Check sheet for the modelled part. Datum: model origin and axes. Units: mm. Give positions to 0.01 mm unless a question says otherwise; leave off trailing zeros. Loops run counter-clockwise (first coordinate to the right, second up) from the corner with the lowest first, then second, coordinate; pieces in that order, holes last. Notation, with made-up numbers: M 22,11.5 L 60,11.5 A10 cw 60,24.5 Z; hole C 26.5,-27 d8. An arc over 180 degrees is marked long. Write each question's results on one line, items separated by ' | '. Start each with the question number.
1. Sectioned sample at C-C on z = 40.64. Record the cut outline in (x, y).
2. Material ranges on line 1 along X through (y, z) = (1.6, 20.32) (3 decimals); line 2 along Z through (x, y) = (1, 4.25); line 3 along X through (y, z) = (2.5, -22) (3 decimals), recorded low to high.
3. Sectioned sample at B-B on y = 1. Record the cut outline in (x, z) (3 decimals), and give its area (3 significant figures).
4. Draft check along Z on faces 1 (the flat face through (-4.696, 3.131, -48.988)), 2 (the cylindrical face through (-2.435, 2.164, -0.767)), 3 (the cylindrical face through (0.553, 2.164, -38.148)), 4 (the flat face through (-4, 0, -1)). Enter one of: pulls with the +Z half, pulls with the -Z half, needs draft (parallel to the pull), parting line crosses it, or undercut.
5. Go/stop test with flat-tipped pins: pin 1 (1 mm diameter, centred on x = 2.5, y = 4, fed in from -Z); pin 2 (1 mm diameter, centred on x = 6, y = 5.5, fed in from -Z). Record where each tip stops, or that it passes through.
6. Sectioned sample at D-D on x = -1. Give the number of separate pieces and of enclosed holes in the cut face, and give its area (3 significant figures).
```python
from build123d import *

# Parameters (mm, degrees)
BOSS_EXTRUDE1_DEPTH                                = 6.35
CSK_FOR_10_FLAT_HEAD_MACHINE_SCREW_100_D           = 5.1054
CSK_FOR_10_FLAT_HEAD_MACHINE_SCREW_100_CSINK_D     = 9.779
CSK_FOR_10_FLAT_HEAD_MACHINE_SCREW_100_CSINK_ANGLE = 100


with BuildPart() as part:
    # Sketch1 → Boss-Extrude1 (new body)
    with BuildSketch(Plane(origin=(0, 0, 0), x_dir=(1, 0, 0), z_dir=(0, 1, 0))):
        Polygon((0, 60.325), (-9.525, 37.329615818), (-9.525, -37.329615818), (0, -60.325), (9.525, -37.329615818), (9.525, 37.329615818), align=None)
    extrude(amount=BOSS_EXTRUDE1_DEPTH)

    # CSK for #10 Flat Head Machine Screw (100)1 (through all)
    with Locations(Plane(origin=(0, 6.35, 0), x_dir=(1, 0, 0), z_dir=(0, 1, 0))):
        with Locations((0, 20.32), (0, 40.64), (0, 0), (0, -20.32), (0, -40.64)):
            CounterSinkHole(CSK_FOR_10_FLAT_HEAD_MACHINE_SCREW_100_D / 2, CSK_FOR_10_FLAT_HEAD_MACHINE_SCREW_100_CSINK_D / 2, counter_sink_angle=CSK_FOR_10_FLAT_HEAD_MACHINE_SCREW_100_CSINK_ANGLE)


solid = part.part
```
Output values:
1) outline: M -8.15,0 L -2.55,0 L -2.55,4.39 L -4.89,6.35 L -8.15,6.35 Z; M 2.55,0 L 8.15,0 L 8.15,6.35 L 4.89,6.35 L 2.55,4.39 Z
2) line 1: -9.525 to -2.553, 2.553 to 9.525 | line 2: -57.91 to -42.99, -38.29 to -22.67, -17.97 to -2.35, 2.35 to 17.97, 22.67 to 38.29, 42.99 to 57.91 | line 3: -9.525 to -1.922, 1.922 to 9.525
3) outline: M -9.525,-37.33 L 0,-60.325 L 9.525,-37.33 L 9.525,37.33 L 0,60.325 L -9.525,37.33 Z; hole C 0,-40.64 d5.105; hole C 0,-20.32 d5.105; hole C 0,0 d5.105; hole C 0,20.32 d5.105; hole C 0,40.64 d5.105 | area: 1,760 mm2
4) face 1: pulls with the -Z half | face 2: undercut | face 3: undercut | face 4: needs draft
5) pin 1: z = -55.5 | pin 2: z = -47.05
6) separate pieces: 6 | enclosed holes: 0 | area: 562 mm2
